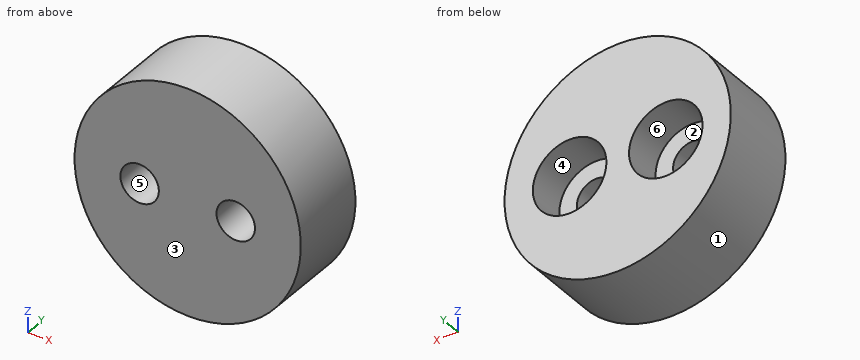
from build123d import *

# Parameters (mm, degrees)
SKIZZE1_R                                            = 10
AUFSATZ_LINEAR_AUSTRAGEN1_DEPTH                      = 7
STIRNSENKUNG_F_R_M3_ZYLINDERSCHRAUBE_MIT_D           = 3.4
STIRNSENKUNG_F_R_M3_ZYLINDERSCHRAUBE_MIT_CBORE_D     = 6.5
STIRNSENKUNG_F_R_M3_ZYLINDERSCHRAUBE_MIT_CBORE_DEPTH = 3.4


with BuildPart() as part:
    # Skizze1 → Aufsatz-Linear austragen1 (new body)
    with BuildSketch(Plane(origin=(0, 0, 0), x_dir=(1, 0, 0), z_dir=(0, 1, 0))):
        with Locations(Location((0, 0, 0), (0, 0, 270))):
            Circle(SKIZZE1_R)
    extrude(amount=AUFSATZ_LINEAR_AUSTRAGEN1_DEPTH)

    # Stirnsenkung für M3 Zylinderschraube mit Innensechskant1 (through all)
    with Locations(Plane(origin=(0, 7, 0), x_dir=(1, 0, 0), z_dir=(0, 1, 0))):
        with Locations((4.25, 0), (-4.25, 0)):
            CounterBoreHole(STIRNSENKUNG_F_R_M3_ZYLINDERSCHRAUBE_MIT_D / 2, STIRNSENKUNG_F_R_M3_ZYLINDERSCHRAUBE_MIT_CBORE_D / 2, STIRNSENKUNG_F_R_M3_ZYLINDERSCHRAUBE_MIT_CBORE_DEPTH)


solid = part.part
Geometry: final body of the model. Coordinates: model frame, mm. Face numbers are marked on the shaded views. A direction names the side the tool comes from. Coordinates: 2 decimals unless noted, no trailing zeros. Loops run counter-clockwise (first coordinate to the right, second up) from the corner with the lowest first, then second, coordinate; pieces in that order, holes last. Notation, with made-up numbers: M 66.5,-19 L 111.5,-19 A24 cw 111.5,9 Z; hole C -37,-24.75 d3. An arc over 180 degrees is marked long. One line per item, written item: value. Start each with the question number.
1) Material intervals for L1, parallel to X at y = 6.5, z = 0.75; L2, parallel to X at y = 4.25, z = 2.5; L3, parallel to Z at x = 4, y = 2.25, sorted ascending. Write a range as from..to.
2) Draft query along Z for the marked faces 1, 2, 3 and 4. Return one class per face: released by +Z, released by -Z, zero draft, split by the parting line, or undercut.
3) Cut plane C-C (y = 5). Return loops of the section in (x, z).
4) Cut plane D-D (x = 3.5). Return loops of the section in (y, z).
5) Cut plane B-B (x = -3). Return loops of the section in (y, z), then the cut area to 3 significant figures.
6) Reachability of the marked faces 5 and 6 from +Z, -Z, +X, -X, +Y, -Y: full face, straight path, thin tool, end or side. Return the list, or none.
7) Cut plane A-A (z = 0). Return loops of the section in (x, y), then the cut area to 3 significant figures.
8) Pin query (flat end, axial travel): P1, Ø1, axis at x = 6.5, y = 5.5, coming from the +Z side; P2, Ø2, axis at y = 6, z = 6.5, coming from the -X side; P3, Ø3, axis at y = 5.5, z = 6.5, coming from the -X side. Return the tip coordinate at first contact, or that it passes through.
Evaluation:
1. L1: -9.97..-7.41, -1.09..1.09, 7.41..9.97
1. L2: -9.68..-6.33, -2.17..2.17, 6.33..9.68
1. L3: -9.17..-1.68, 1.68..9.17
2. face 1: split by the parting line
2. face 2: undercut
2. face 3: zero draft
2. face 4: undercut
3. outline: C 0,0 d20; hole C -4.25,0 d6.5; hole C 4.25,0 d6.5
4. outline: M 0,-9.37 L 7,-9.37 L 7,-3.16 L 3.6,-3.16 L 3.6,-1.53 L 0,-1.53 Z; M 0,1.53 L 3.6,1.53 L 3.6,3.16 L 7,3.16 L 7,9.37 L 0,9.37 Z
5. outline: M 0,-9.54 L 7,-9.54 L 7,-3 L 3.6,-3 L 3.6,-1.15 L 0,-1.15 Z; M 0,1.15 L 3.6,1.15 L 3.6,3 L 7,3 L 7,9.54 L 0,9.54 Z
5. area: 105 mm^2
6. face 5: +Y, -Y
6. face 6: +Y
7. outline: M -10,0 L -5.95,0 L -5.95,3.6 L -7.5,3.6 L -7.5,7 L -10,7 Z; M -2.55,0 L 2.55,0 L 2.55,3.6 L 1,3.6 L 1,7 L -1,7 L -1,3.6 L -2.55,3.6 Z; M 5.95,0 L 10,0 L 10,7 L 7.5,7 L 7.5,3.6 L 5.95,3.6 Z
7. area: 71.3 mm^2
8. P1: z = 8
8. P2: x = -8.35
8. P3: x = -8.66
